```python
from build123d import *

# Parameters (mm, degrees)
SKETCH1_W           = 15.9
SKETCH1_H           = 7.95
BOSS_EXTRUDE1_DEPTH = 7.95
SKETCH2_R           = 2.4
BOSS_EXTRUDE2_DEPTH = 1.8
LPATTERN1_COUNT     = 2
LPATTERN1_PITCH     = 8
SHELL1_T            = -1.2


with BuildPart() as part:
    # Sketch1 → Boss-Extrude1 (new body)
    with BuildSketch(Plane.XY):
        Rectangle(SKETCH1_W, SKETCH1_H)
    extrude(amount=-BOSS_EXTRUDE1_DEPTH)

    # Sketch2 → Boss-Extrude2 (add)
    with BuildSketch(Plane(origin=(0, 3.975, 0), x_dir=(1, 0, 0), z_dir=(0, 1, 0))):
        with Locations(Location((-4.05, 3.9, 0), (0, 0, 270))):
            Circle(SKETCH2_R)
    boss_extrude2 = extrude(amount=BOSS_EXTRUDE2_DEPTH)

    # LPattern1: Boss-Extrude2 ×2
    with Locations(*[(i * LPATTERN1_PITCH, 0, 0) for i in range(1, LPATTERN1_COUNT)]):
        add(boss_extrude2)

    # Shell1
    shell1_openings = [part.faces().sort_by_distance(p)[0] for p in [
        (0, -3.975, -3.975),
    ]]
    offset(amount=SHELL1_T, openings=shell1_openings, kind=Kind.INTERSECTION)


solid = part.part
```
The listing builds one solid part. Answer for the finished solid, in the listing's coordinates (mm). A direction names the side the tool comes from. Round coordinates to 2 decimals unless told otherwise and drop trailing zeros. Order: outer loops, then holes, each group sorted by start corner. A loop starts at its lowest first (then second) coordinate and runs counter-clockwise, first axis right, second up. Notation, with made-up numbers: (87, 74.25) -> (110, 74.25) arc R11 cw to (110, 92.25) -> close; hole circle Ø1 at (0.25, 67). An arc over 180 degrees is marked (long way). Answer as CSV lines item,"result".
Q1. A cutting plane is placed at C-C on z = -3.9. Determine the outline of the cut face in (x, y) (3 decimals).
Computed values:
outline,"(-7.95, -3.975) -> (-6.75, -3.975) -> (-6.75, 2.775) -> (-5.25, 2.775) -> (-5.25, 4.575) -> (-2.85, 4.575) -> (-2.85, 2.775) -> (2.75, 2.775) -> (2.75, 4.575) -> (5.15, 4.575) -> (5.15, 2.775) -> (6.75, 2.775) -> (6.75, -3.975) -> (7.95, -3.975) -> (7.95, 3.975) -> (6.35, 3.975) -> (6.35, 5.775) -> (1.55, 5.775) -> (1.55, 3.975) -> (-1.65, 3.975) -> (-1.65, 5.775) -> (-6.45, 5.775) -> (-6.45, 3.975) -> (-7.95, 3.975) -> close"
Q2. Consider line 1 (X direction, y = 3.5, z = -3.9); line 2 (Z direction, x = -4.05, y = 3.4); line 3 (Z direction, x = 3.5, y = 1.5). Determine where each line is inside the solid, lowest interval first. Write a range as from..to.
Computed values:
line 1,"x = -7.95..-5.25, -2.85..2.75, 5.15..7.95"
line 2,"z = -7.95..-5.1, -2.7..0"
line 3,"z = -7.95..-6.75, -1.2..0"
Q3. Given pin 1 (1.2 mm diameter, centred on x = -4, z = -3.5, fed in from -Y) (3 decimals); pin 2 (3 mm diameter, centred on x = 0, z = -5, fed in from +Y) (3 decimals), each flat-ended and moving along its own axis, determine where each tip first touches the part or whether it passes through.
Computed values:
pin 1,"stops at y = 4.575"
pin 2,"stops at y = 3.975"
Q4. A cutting plane is placed at A-A on y = -0.5. Determine the outline of the cut face in (x, z), plus the area to 3 significant figures.
Computed values:
outline,"(-7.95, -7.95) -> (7.95, -7.95) -> (7.95, 0) -> (-7.95, 0) -> close; hole (-6.75, -6.75) -> (6.75, -6.75) -> (6.75, -1.2) -> (-6.75, -1.2) -> close"
area,"51.5 mm^2"
Q5. Which of the six approach directions +Z, -Z, +X, -X, +Y, -Y give full straight-line access (tool end or side, diameter ignored) to faces 4 (the flat face through (4, 5.775, -4)), 5 (the flat face through (-6.75, -1, -4)), 6 (the flat face through (0, 3.975, -4))?
Computed values:
face 4,"+Z, -Z, +X, -X, +Y"
face 5,"-Y"
face 6,"+Y"
Q6. A cutting plane is placed at D-D on z = -6.5. Determine the outline of the cut face in (x, y) (3 decimals), plus the area to 3 significant figures.
Computed values:
outline,"(-7.95, -3.975) -> (-6.75, -3.975) -> (-6.75, 2.775) -> (6.75, 2.775) -> (6.75, -3.975) -> (7.95, -3.975) -> (7.95, 3.975) -> (-7.95, 3.975) -> close"
area,"35.3 mm^2"
Q7. For a pull along Z with two mould halves and no side action, classify faces 1 (the flat face through (0, -3.975, -7)), 2 (the flat face through (0, 0, 0)), 3 (the flat face through (6.75, -1, -4)) as +Z half, -Z half, draft (parallel to the pull), parting line (faces both ways), or undercut.
Computed values:
face 1,"draft"
face 2,"+Z half"
face 3,"undercut"
Q8. A cutting plane is placed at B-B on x = 3.95. Determine the outline of the cut face in (y, z) (3 decimals), plus the area to 3 significant figures.
Computed values:
outline,"(-3.975, -7.95) -> (3.975, -7.95) -> (3.975, -6.3) -> (5.775, -6.3) -> (5.775, -1.5) -> (3.975, -1.5) -> (3.975, 0) -> (-3.975, 0) -> (-3.975, -1.2) -> (2.775, -1.2) -> (2.775, -2.7) -> (4.575, -2.7) -> (4.575, -5.1) -> (2.775, -5.1) -> (2.775, -6.75) -> (-3.975, -6.75) -> close"
area,"30.1 mm^2"
